from build123d import *

# Parameters (mm, degrees)
SKETCH_1_W          = 9
SKETCH_1_H          = 6.5
EXTRUDE_1_DEPTH     = 510
SKETCH_2_W          = 2
SKETCH_2_H          = 1
CUT_EXTRUDE_1_DEPTH = 450
SKETCH_3_R          = 1.5
CUT_EXTRUDE_2_DEPTH = 6.5


with BuildPart() as part:
    # 草图1 → 凸台-拉伸1 (new body)
    with BuildSketch(Plane.XY):
        with Locations((-4.5, 3.25)):
            Rectangle(SKETCH_1_W, SKETCH_1_H)
    extrude(amount=EXTRUDE_1_DEPTH)

    # 草图2 → 切除-拉伸1 (cut)
    with BuildSketch(Plane(origin=(0, 0, 0), x_dir=(-1, 0, 0), z_dir=(0, 0, -1))):
        with Locations((1, 5)):
            Rectangle(SKETCH_2_W, SKETCH_2_H)
        with Locations((8, 5)):
            Rectangle(SKETCH_2_W, SKETCH_2_H)
    extrude(amount=-CUT_EXTRUDE_1_DEPTH, mode=Mode.SUBTRACT)

    # 草图3 → 切除-拉伸2 (cut)
    with BuildSketch(Plane(origin=(0, 6.5, 0), x_dir=(1, 0, 0), z_dir=(0, 1, 0))):
        with Locations(Location((-4.5, -5, 0), (0, 0, 180))):
            Circle(SKETCH_3_R)
        with Locations(Location((-4.5, -25, 0), (0, 0, 180))):
            Circle(SKETCH_3_R)
        with Locations(Location((-4.5, -45, 0), (0, 0, 180))):
            Circle(SKETCH_3_R)
        with Locations(Location((-4.5, -65, 0), (0, 0, 180))):
            Circle(SKETCH_3_R)
        with Locations(Location((-4.5, -85, 0), (0, 0, 180))):
            Circle(SKETCH_3_R)
        with Locations(Location((-4.5, -105, 0), (0, 0, 180))):
            Circle(SKETCH_3_R)
        with Locations(Location((-4.5, -125, 0), (0, 0, 180))):
            Circle(SKETCH_3_R)
        with Locations(Location((-4.5, -145, 0), (0, 0, 180))):
            Circle(SKETCH_3_R)
        with Locations(Location((-4.5, -165, 0), (0, 0, 180))):
            Circle(SKETCH_3_R)
        with Locations(Location((-4.5, -185, 0), (0, 0, 180))):
            Circle(SKETCH_3_R)
        with Locations(Location((-4.5, -205, 0), (0, 0, 180))):
            Circle(SKETCH_3_R)
        with Locations(Location((-4.5, -225, 0), (0, 0, 180))):
            Circle(SKETCH_3_R)
        with Locations(Location((-4.5, -245, 0), (0, 0, 180))):
            Circle(SKETCH_3_R)
        with Locations(Location((-4.5, -265, 0), (0, 0, 180))):
            Circle(SKETCH_3_R)
        with Locations(Location((-4.5, -285, 0), (0, 0, 180))):
            Circle(SKETCH_3_R)
        with Locations(Location((-4.5, -305, 0), (0, 0, 180))):
            Circle(SKETCH_3_R)
        with Locations(Location((-4.5, -325, 0), (0, 0, 180))):
            Circle(SKETCH_3_R)
        with Locations(Location((-4.5, -345, 0), (0, 0, 180))):
            Circle(SKETCH_3_R)
        with Locations(Location((-4.5, -365, 0), (0, 0, 180))):
            Circle(SKETCH_3_R)
        with Locations(Location((-4.5, -385, 0), (0, 0, 180))):
            Circle(SKETCH_3_R)
        with Locations(Location((-4.5, -405, 0), (0, 0, 180))):
            Circle(SKETCH_3_R)
        with Locations(Location((-4.5, -425, 0), (0, 0, 180))):
            Circle(SKETCH_3_R)
        with Locations(Location((-4.5, -445, 0), (0, 0, 180))):
            Circle(SKETCH_3_R)
        with Locations(Location((-4.5, -465, 0), (0, 0, 180))):
            Circle(SKETCH_3_R)
        with Locations(Location((-4.5, -485, 0), (0, 0, 180))):
            Circle(SKETCH_3_R)
        with Locations(Location((-4.5, -505, 0), (0, 0, 180))):
            Circle(SKETCH_3_R)
    extrude(amount=-CUT_EXTRUDE_2_DEPTH, mode=Mode.SUBTRACT)


solid = part.part
Geometry check sheet. Reference: the model listing, model coordinates, mm. Give positions to 0.01 mm unless a question says otherwise; leave off trailing zeros. Loops run counter-clockwise (first coordinate to the right, second up) from the corner with the lowest first, then second, coordinate; pieces in that order, holes last. Notation, with made-up numbers: (-9.5, -37) -> (44.5, -37) arc R8 ccw to (44.5, -24) -> close; hole circle Ø7 at (43, -33.5). An arc over 180 degrees is marked (long way). Answer in a Markdown table with one row per item. Add a question column.
1) Cross-section at A-A on y = 1.5. State how many separate pieces and enclosed holes the cut face has, and give its area (3 significant figures).
2) Cross-section at B-B on z = 234. Record the boundary of the cut face in (x, y), and give its area (3 significant figures).
3) Material ranges on probe 1 along Y at (x, z) = (-7.5, 37); probe 2 along X at (y, z) = (2.75, 205); probe 3 along X at (y, z) = (5.25, 337), recorded low to high. Write a range as from..to.
Outcome:
| question | item | result |
|---|---|---|
| 1 | separate pieces | 1 |
| 1 | enclosed holes | 26 |
| 1 | area | 4,410 mm^2 |
| 2 | outline | (-9, 0) -> (0, 0) -> (0, 4.5) -> (-2, 4.5) -> (-2, 5.5) -> (0, 5.5) -> (0, 6.5) -> (-9, 6.5) -> (-9, 5.5) -> (-7, 5.5) -> (-7, 4.5) -> (-9, 4.5) -> close |
| 2 | area | 54.5 mm^2 |
| 3 | probe 1 | y = 0..4.5, 5.5..6.5 |
| 3 | probe 2 | x = -9..-6, -3..0 |
| 3 | probe 3 | x = -7..-2 |
